Check sheet for the modelled part. Datum: model origin and axes. Units: mm. A direction names the side the tool comes from. Coordinates: 2 decimals unless noted, no trailing zeros. Order: outer loops, then holes, each group sorted by start corner. A loop starts at its lowest first (then second) coordinate and runs counter-clockwise, first axis right, second up.
1. Cross-section at B-B (x = 0). Enter the section's corners in (y, z).
2. Draft check along X on faces 1 (the flat face through (2, 1, 1)), 2 (the flat face through (-36.5, -3, 1)), 3 (the flat face through (5, 0, 1)). Enter one of: released by +X, released by -X, zero draft, split by the parting line, or undercut.
3. Cross-section at D-D (x = -15). Enter the section's corners in (y, z).
4. Thickness scan on line 1 (X direction, y = -12.75, z = 5.5); line 2 (Y direction, x = 29, z = -0.5); line 3 (Y direction, x = 17.5, z = 7.25). Record the ranges inside material, lowest first.
5. Gauge pin test, flat ends, axial feed: pin 1 Ø1.6 at (x, z) = (13.5, 5) entering from +Y; pin 2 Ø0.5 at (y, z) = (0.5, 4.5) entering from -X; pin 3 Ø5 at (x, z) = (24, 2.5) entering from -Y; pin 4 Ø2.5 at (y, z) = (-10, 7.5) entering from +X. Record the tip position at first contact, or that the pin passes through.
6. Set-up check for faces 4 (the flat face through (4, -15, 7)), 5 (the flat face through (0, -9, 4.46)), 6 (the flat face through (-18, 0, 1)): record each of +Z, -Z, +X, -X, +Y, -Y from which the full face is reachable in a straight line by a thin tool's end or side.
7. Cross-section at C-C (y = -7). Enter the section's corners in (x, z), then the cut area to 3 significant figures.
8. Cross-section at A-A (y = -11.25). Enter the section's corners in (x, z).
```python
from build123d import *

# Parameters (mm, degrees)
SKETCH4_W            = 73
SKETCH4_H            = 15
BOSS_EXTRUDE4_DEPTH  = 6
SKETCH15_W           = 3
SKETCH15_H           = 15
BOSS_EXTRUDE6_DEPTH  = 1
BOSS_EXTRUDE7_DEPTH  = 1.5
BOSS_EXTRUDE13_DEPTH = 7.715
CUT_EXTRUDE2_REACH   = 40.656
SKETCH22_W           = 12
SKETCH22_H           = 3.715
CUT_EXTRUDE3_REACH   = 42.428
BOSS_EXTRUDE14_DEPTH = 2.54


with BuildPart() as part:
    # Sketch4 → Boss-Extrude4 (new body)
    with BuildSketch(Plane(origin=(0, 0, 0), x_dir=(-1, 0, 0), z_dir=(0, 1, 0))):
        Rectangle(SKETCH4_W, SKETCH4_H)
    extrude(amount=-BOSS_EXTRUDE4_DEPTH)

    # Sketch15 → Boss-Extrude6 (add)
    with BuildSketch(Plane(origin=(0, 0, 0), x_dir=(1, 0, 0), z_dir=(0, 1, 0))):
        with Locations((2.25, 0)):
            Rectangle(SKETCH15_W, SKETCH15_H)
        with Locations((6.75, 0)):
            Rectangle(SKETCH15_W, SKETCH15_H)
        with Locations((11.25, 0)):
            Rectangle(SKETCH15_W, SKETCH15_H)
        with Locations((15.75, 0)):
            Rectangle(SKETCH15_W, SKETCH15_H)
        with Locations((20.25, 0)):
            Rectangle(SKETCH15_W, SKETCH15_H)
        with Locations((24.75, 0)):
            Rectangle(SKETCH15_W, SKETCH15_H)
        with Locations((29.25, 0)):
            Rectangle(SKETCH15_W, SKETCH15_H)
        with Locations((33.75, 0)):
            Rectangle(SKETCH15_W, SKETCH15_H)
        with Locations((-33.75, 0)):
            Rectangle(SKETCH15_W, SKETCH15_H)
        with Locations((-29.25, 0)):
            Rectangle(SKETCH15_W, SKETCH15_H)
        with Locations((-24.75, 0)):
            Rectangle(SKETCH15_W, SKETCH15_H)
        with Locations((-20.25, 0)):
            Rectangle(SKETCH15_W, SKETCH15_H)
        with Locations((-15.75, 0)):
            Rectangle(SKETCH15_W, SKETCH15_H)
        with Locations((-11.25, 0)):
            Rectangle(SKETCH15_W, SKETCH15_H)
        with Locations((-6.75, 0)):
            Rectangle(SKETCH15_W, SKETCH15_H)
        with Locations((-2.25, 0)):
            Rectangle(SKETCH15_W, SKETCH15_H)
    extrude(amount=BOSS_EXTRUDE6_DEPTH)

    # Sketch16 → Boss-Extrude7 (add)
    with BuildSketch(Plane.XY.offset(7.5)):
        Polygon((-35.25, 0), (-36.5, 0), (-36.5, -6), (36.5, -6), (36.5, 0), (35.25, 0), (35.25, 1), (32.25, 1), (32.25, 0), (30.75, 0), (30.75, 1), (27.75, 1), (27.75, 0), (26.25, 0), (26.25, 1), (23.25, 1), (23.25, 0), (21.75, 0), (21.75, 1), (18.75, 1), (18.75, 0), (17.25, 0), (17.25, 1), (14.25, 1), (14.25, 0), (12.75, 0), (12.75, 1), (9.75, 1), (9.75, 0), (8.25, 0), (8.25, 1), (5.25, 1), (5.25, 0), (3.75, 0), (3.75, 1), (0.75, 1), (0.75, 0), (-0.75, 0), (-0.75, 1), (-3.75, 1), (-3.75, 0), (-5.25, 0), (-5.25, 1), (-8.25, 1), (-8.25, 0), (-9.75, 0), (-9.75, 1), (-12.75, 1), (-12.75, 0), (-14.25, 0), (-14.25, 1), (-17.25, 1), (-17.25, 0), (-18.75, 0), (-18.75, 1), (-21.75, 1), (-21.75, 0), (-23.25, 0), (-23.25, 1), (-26.25, 1), (-26.25, 0), (-27.75, 0), (-27.75, 1), (-30.75, 1), (-30.75, 0), (-32.25, 0), (-32.25, 1), (-35.25, 1), align=None)
    extrude(amount=BOSS_EXTRUDE7_DEPTH)

    # Sketch21 → Boss-Extrude13 (add)
    with BuildSketch(Plane.XY.offset(9)):
        with BuildLine():
            Line((-2.54, -12), (-2.54, -15))
            Line((-2.54, -15), (-6, -15))
            Line((-6, -15), (-6, -6))
            Line((-6, -6), (6, -6))
            Line((6, -6), (6, -15))
            Line((6, -15), (2.54, -15))
            Line((2.54, -15), (2.54, -12))
            ThreePointArc((2.54, -12), (0, -9.46), (-2.54, -12))
        make_face()
    extrude(amount=-BOSS_EXTRUDE13_DEPTH)

    # Cut-Extrude2: up to this face of the body (flat: up to its plane)
    cut_extrude2_end = Plane(part.part.faces().sort_by_distance((4.27, -15, 5.1425))[0])
    # Sketch22 → Cut-Extrude2 (cut, up to the picked face)
    with BuildSketch(Plane.XZ.offset(6), mode=Mode.PRIVATE) as cut_extrude2_sk1:
        with Locations((0, 5.1425)):
            Rectangle(SKETCH22_W, SKETCH22_H)
    cut_extrude2_tool1 = split(extrude(cut_extrude2_sk1.sketch, amount=CUT_EXTRUDE2_REACH, mode=Mode.PRIVATE), bisect_by=cut_extrude2_end, keep=Keep.BOTH, mode=Mode.PRIVATE)
    add(cut_extrude2_tool1.solids().sort_by(Axis((0, -6, 5.1425), (0, -1, 0)))[0], mode=Mode.SUBTRACT)

    # Sketch23 → Cut-Extrude3 (cut, up to next)
    with BuildSketch(Plane(origin=(0, 0, 1.285), x_dir=(-1, 0, 0), z_dir=(0, 0, -1)), mode=Mode.PRIVATE) as cut_extrude3_sk1:
        with BuildLine():
            Line((6, -15), (6, -6))
            Line((6, -6), (-6, -6))
            Line((-6, -6), (-6, -15))
            Line((-6, -15), (-2.54, -15))
            Line((-2.54, -15), (-2.54, -12))
            ThreePointArc((-2.54, -12), (0, -9.46), (2.54, -12))
            Line((2.54, -12), (2.54, -15))
            Line((2.54, -15), (6, -15))
        make_face()
    cut_extrude3_tool1 = extrude(cut_extrude3_sk1.sketch, amount=-CUT_EXTRUDE3_REACH, mode=Mode.PRIVATE) & part.part
    add(cut_extrude3_tool1.solids().sort_by_distance((-5.85, -10.5, 1.285))[0], mode=Mode.SUBTRACT)

    # Sketch24 → Boss-Extrude14 (add)
    with BuildSketch(Plane(origin=(0, 0, 7), x_dir=(-1, 0, 0), z_dir=(0, 0, -1))):
        with BuildLine():
            Line((2.54, -12), (2.54, -15))
            Line((2.54, -15), (6, -15))
            Line((6, -15), (6, -6))
            Line((6, -6), (-6, -6))
            Line((-6, -6), (-6, -15))
            Line((-6, -15), (-2.54, -15))
            Line((-2.54, -15), (-2.54, -12))
            ThreePointArc((-2.54, -12), (0, -9.46), (2.54, -12))
        make_face()
    extrude(amount=BOSS_EXTRUDE14_DEPTH)


solid = part.part
```
Data:
1. outline: (-9.46, 4.46) - (-6, 4.46) - (-6, -7.5) - (0, -7.5) - (0, 9) - (-9.46, 9) - close
2. face 1: zero draft
2. face 2: released by -X
2. face 3: undercut
3. outline: (-6, -7.5) - (1, -7.5) - (1, 9) - (-6, 9) - close
4. line 1: x = -6 to -2.54, 2.54 to 6
4. line 2: y = -6 to 1
4. line 3: y = -6 to 0
5. pin 1: stops at y = 1
5. pin 2: stops at x = -35.25
5. pin 3: stops at y = -6
5. pin 4: stops at x = 6
6. face 4: +Z, -Z, +X, -X, -Y
6. face 5: -Z, +X, -X, -Y
6. face 6: +Z, -Z, +Y
7. outline: (-6, 4.46) - (6, 4.46) - (6, 9) - (-6, 9) - close
7. area: 54.5 mm2
8. outline: (-6, 4.46) - (-2.43, 4.46) - (-2.43, 9) - (-6, 9) - close; (2.43, 4.46) - (6, 4.46) - (6, 9) - (2.43, 9) - close
